Build history of the part. All positions in model axes, mm. Round coordinates to 2 decimals unless told otherwise and drop trailing zeros. Order: outer loops, then holes, each group sorted by start corner. A loop starts at its lowest first (then second) coordinate and runs counter-clockwise, first axis right, second up. Notation, with made-up numbers: (25.25, 31.25) - (63.25, 31.25) arc R19 ccw to (63.25, 62.25) - close; hole circle Ø2 at (89, 69). An arc over 180 degrees is marked (long way). Write each question's results on one line, items separated by ' | '. Start each with the question number.
```python
from build123d import *

# Parameters (mm, degrees)
SKETCH_1_W          = 26
SKETCH_1_H          = 23
EXTRUDE_1_DEPTH     = 3
CHAMFER_1_SIZE      = 1.5
CUT_EXTRUDE_1_DEPTH = 4
CHAMFER_2_SIZE      = 1


with BuildPart() as part:
    # Эскиз1 → Вытянуть1 (new body)
    with BuildSketch(Plane.XY):
        with Locations((0, 1.5)):
            Rectangle(SKETCH_1_W, SKETCH_1_H)
    extrude(amount=EXTRUDE_1_DEPTH)

    # Фаска1
    chamfer_1_edges = [part.edges().sort_by_distance(p)[0] for p in [
        (0, -10, 3),
    ]]
    chamfer(chamfer_1_edges, length=CHAMFER_1_SIZE)

    # Эскиз2 → Вырез-Вытянуть1 (cut, through all)
    with BuildSketch(Plane(origin=(0, 0, 0), x_dir=(-1, 0, 0), z_dir=(0, 0, -1))):
        Polygon((-81.137767415, 0), (-13, 0), (-4, 0), (-4, -10), (-4, -78.137767415), (-100.979926637, -173.876553822), (-178.117694052, -95.738786407), align=None)
    extrude(amount=-CUT_EXTRUDE_1_DEPTH, mode=Mode.SUBTRACT)

    # Фаска2
    chamfer_2_edges = [part.edges().sort_by_distance(p)[0] for p in [
        (0, 13, 3),
        (8.5, 0, 3),
    ]]
    chamfer(chamfer_2_edges, length=CHAMFER_2_SIZE)


solid = part.part
```
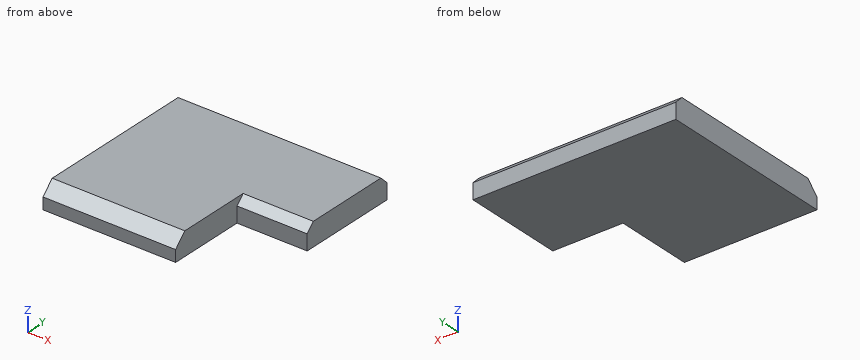
1. Cut at A-A (z = 2.55). List the corners of the cut face in (x, y), plus the area to 3 significant figures.
2. Wall check: line 1 (X direction, y = -5, z = 2.1); line 2 (Y direction, x = 4.25, z = 1.5); line 3 (Y direction, x = -11.5, z = 1.8). Give the ranges that are in metal, low to high. Write a range as from..to.
3. Cut at B-B (x = 8.25). List the corners of the cut face in (y, z), plus the area to 3 significant figures.
4. Cut at C-C (y = -7). List the corners of the cut face in (x, z).
5. Flat gauge pins, fed straight in: pin 1 Ø0.6 at (x, z) = (8.5, 1) entering from -Y; pin 2 Ø1.5 at (y, z) = (-2.5, 2) entering from +X; pin 3 Ø1.5 at (x, y) = (7, -1.5) entering from -Z. Where does each tip first touch, or does it go through?
A:
1) outline: (-13, -8.95) - (4, -8.95) - (4, 0.55) - (13, 0.55) - (13, 12.45) - (-13, 12.45) - close | area: 471 mm^2
2) line 1: x = -13..4 | line 2: y = 0..13 | line 3: y = -9.7..13
3) outline: (0, 0) - (13, 0) - (13, 2) - (12, 3) - (1, 3) - (0, 2) - close | area: 38.0 mm^2
4) outline: (-13, 0) - (4, 0) - (4, 3) - (-13, 3) - close
5) pin 1: stops at y = 0 | pin 2: stops at x = 4 | pin 3: passes through
